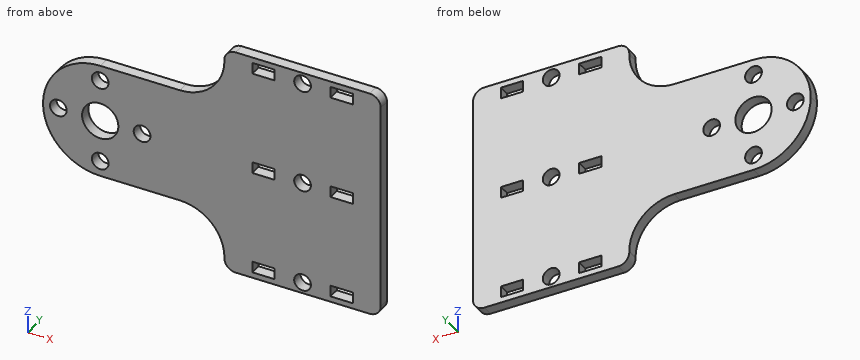
```python
from build123d import *

# Parameters (mm, degrees)
SKETCH1_R           = 3.25
SKETCH1_R_2         = 1.5
BOSS_EXTRUDE1_DEPTH = 2
FILLET1_R           = 10.25
FILLET2_R           = 2
SKETCH2_R           = 1.5
SKETCH2_W           = 4
SKETCH2_H           = 2
CUT_EXTRUDE1_DEPTH  = 2
FILLET3_R           = 8


with BuildPart() as part:
    # Sketch1 → Boss-Extrude1 (new body)
    with BuildSketch(Plane(origin=(0, 0, 0), x_dir=(1, 0, 0), z_dir=(0, 1, 0))):
        Polygon((0, 0), (32.5, 0), (32.5, -10.25), (60.5, -10.25), (60.5, -0.75), (60.5, 21.25), (60.5, 30.75), (32.5, 30.75), (32.5, 20.5), (0, 20.5), align=None)
        with Locations(Location((10.25, 10.25, 0), (0, 0, 270))):
            Circle(SKETCH1_R, mode=Mode.SUBTRACT)
        with Locations(Location((2.75, 10.25, 0), (0, 0, 270))):
            Circle(SKETCH1_R_2, mode=Mode.SUBTRACT)
        with Locations(Location((10.25, 17.75, 0), (0, 0, 90))):
            Circle(SKETCH1_R_2, mode=Mode.SUBTRACT)
        with Locations(Location((17.75, 10.25, 0), (0, 0, 270))):
            Circle(SKETCH1_R_2, mode=Mode.SUBTRACT)
        with Locations(Location((10.25, 2.75, 0), (0, 0, 90))):
            Circle(SKETCH1_R_2, mode=Mode.SUBTRACT)
    extrude(amount=BOSS_EXTRUDE1_DEPTH)

    # Fillet1
    fillet1_edges = [part.edges().sort_by_distance(p)[0] for p in [
        (0, 1, -20.5),
        (0, 1, 0),
    ]]
    fillet(fillet1_edges, radius=FILLET1_R - 0.0001)  # a hair under: the kernel refuses the full size

    # Fillet2
    fillet2_edges = [part.edges().sort_by_distance(p)[0] for p in [
        (32.5, 1, -30.75),
        (60.5, 1, -30.75),
        (60.5, 1, 10.25),
        (32.5, 1, 10.25),
    ]]
    fillet(fillet2_edges, radius=FILLET2_R)

    # Sketch2 → Cut-Extrude1 (cut)
    with BuildSketch(Plane(origin=(0, 2, 0), x_dir=(1, 0, 0), z_dir=(0, 1, 0))):
        with Locations(Location((46.5, 28.75, 0), (0, 0, 270))):
            Circle(SKETCH2_R)
        with Locations(Location((46.5, 10.25, 0), (0, 0, 270))):
            Circle(SKETCH2_R)
        with Locations(Location((46.5, -8.25, 0), (0, 0, 270))):
            Circle(SKETCH2_R)
        with Locations((39.5, 28.75)):
            Rectangle(SKETCH2_W, SKETCH2_H)
        with Locations((53.5, 28.75)):
            Rectangle(SKETCH2_W, SKETCH2_H)
        with Locations((39.5, 10.25)):
            Rectangle(SKETCH2_W, SKETCH2_H)
        with Locations((53.5, 10.25)):
            Rectangle(SKETCH2_W, SKETCH2_H)
        with Locations((39.5, -8.25)):
            Rectangle(SKETCH2_W, SKETCH2_H)
        with Locations((53.5, -8.25)):
            Rectangle(SKETCH2_W, SKETCH2_H)
    extrude(amount=-CUT_EXTRUDE1_DEPTH, mode=Mode.SUBTRACT)

    # Fillet3
    fillet3_edges = [part.edges().sort_by_distance(p)[0] for p in [
        (32.5, 1, -20.5),
        (32.5, 1, 0),
    ]]
    fillet(fillet3_edges, radius=FILLET3_R)


solid = part.part
```
Model file for the job. Use its own axes, mm. Round coordinates to 2 decimals unless told otherwise and drop trailing zeros. Write each loop counter-clockwise with the first axis right and the second up, starting at its lowest first coordinate (ties: lowest second). Pieces come first, ordered by that corner, then holes. Notation, with made-up numbers: (40, 13.25) - (82, 13.25) arc R19 cw to (82, 41.25) - close; hole circle Ø6 at (61.5, 50.5). An arc over 180 degrees is marked (long way). Use CSV: the item, a comma, the result in double quotes. Start each with the question number.
Item 1: Drill centre lines: L1, parallel to Z at x = 38, y = 1.6; L2, parallel to X at y = 1.5, z = 8.25; L3, parallel to X at y = 1.2, z = -11.5. Where is each one in solid material? Low to high. Write a range as [from, to].
Item 2: Band-saw the part on A-A (x = 2.75). Write the cut outline in (y, z).
Item 3: Band-saw the part on C-C (y = 0.7). State how many separate pieces and enclosed holes the cut face has, and give its area (3 significant figures).
Item 4: Band-saw the part on B-B (z = -17.75). Write the cut outline in (x, y), and give its area (3 significant figures).
Item 5: Band-saw the part on D-D (x = 20). Write the cut outline in (y, z), and give its area (3 significant figures).
Checked values:
1,L1,"z = [-30.75, -29.75], [-27.75, -11.25], [-9.25, 7.25], [9.25, 10.25]"
1,L2,"x = [32.5, 37.5], [41.5, 45], [48, 51.5], [55.5, 60.5]"
1,L3,"x = [0.08, 1.92], [3.58, 7.25], [13.25, 16.92], [18.58, 45.67], [47.33, 60.5]"
2,outline,"(0, -17.24) - (2, -17.24) - (2, -11.75) - (0, -11.75) - close; (0, -8.75) - (2, -8.75) - (2, -3.26) - (0, -3.26) - close"
3,separate pieces,"1"
3,enclosed holes,"14"
3,area,"1,660 mm²"
4,outline,"(3.26, 0) - (8.75, 0) - (8.75, 2) - (3.26, 2) - close; (11.75, 0) - (60.5, 0) - (60.5, 2) - (11.75, 2) - close"
4,area,"108 mm²"
5,outline,"(0, -20.5) - (2, -20.5) - (2, 0) - (0, 0) - close"
5,area,"41.0 mm²"
